```python
from build123d import *

# Parameters (mm, degrees)
BOX268_W                    = 56.5
BOX268_H                    = 56.5
BOX268_DEPTH                = 2
CYLINDER687_R               = 1.5
CYLINDER687_DEPTH           = 20
CYLINDER686_R               = 1.5
CYLINDER686_DEPTH           = 20
COMPOUND411_PLACEMENT_ANGLE = 90
BOX266_W                    = 20
BOX266_H                    = 8
BOX266_DEPTH                = 3
BOX265_W                    = 20
BOX265_H                    = 8
BOX265_DEPTH                = 3
BOX267_W                    = 20
BOX267_H                    = 8
BOX267_DEPTH                = 3
BOX264_W                    = 20
BOX264_H                    = 8
BOX264_DEPTH                = 3
CYLINDER682_R               = 12
CYLINDER682_DEPTH           = 20
CYLINDER672_R               = 5
CYLINDER672_DEPTH           = 4
CYLINDER670_R               = 5
CYLINDER670_DEPTH           = 4
CYLINDER674_R               = 5
CYLINDER674_DEPTH           = 4
CYLINDER675_R               = 5
CYLINDER675_DEPTH           = 4
CYLINDER683_R               = 2.5
CYLINDER683_DEPTH           = 20
CYLINDER673_R               = 2.5
CYLINDER673_DEPTH           = 20
CYLINDER676_R               = 2.5
CYLINDER676_DEPTH           = 20
CYLINDER684_R               = 2.5
CYLINDER684_DEPTH           = 20
CYLINDER681_R               = 3
CYLINDER681_DEPTH           = 5
CYLINDER681_PLACEMENT_ANGLE = 22.5
CYLINDER669_R               = 3
CYLINDER669_DEPTH           = 5
CYLINDER669_PLACEMENT_ANGLE = 67.5
CYLINDER680_R               = 3
CYLINDER680_DEPTH           = 5
CYLINDER680_PLACEMENT_ANGLE = 202.5
CYLINDER677_R               = 3
CYLINDER677_DEPTH           = 5
CYLINDER677_PLACEMENT_ANGLE = 112.5
COMPOUND408_PLACEMENT_ANGLE = 45
CYLINDER679_R               = 1.5
CYLINDER679_DEPTH           = 30
CYLINDER679_PLACEMENT_ANGLE = 22.5
CYLINDER678_R               = 1.5
CYLINDER678_DEPTH           = 30
CYLINDER678_PLACEMENT_ANGLE = 67.5
CYLINDER685_R               = 1.5
CYLINDER685_DEPTH           = 30
CYLINDER685_PLACEMENT_ANGLE = 202.5
CYLINDER671_R               = 1.5
CYLINDER671_DEPTH           = 30
CYLINDER671_PLACEMENT_ANGLE = 112.5
COMPOUND409_PLACEMENT_ANGLE = 45
BOX263_W                    = 68
BOX263_H                    = 64
BOX263_DEPTH                = 8


with BuildPart() as krychle268:
    # Box268 → Box268 (new body)
    with BuildSketch(Plane(origin=(-28.25, -28.25, -68), x_dir=(1, 0, 0), z_dir=(0, 0, 1))):
        with Locations((28.25, 28.25)):
            Rectangle(BOX268_W, BOX268_H)
    extrude(amount=BOX268_DEPTH)


with BuildPart() as obj1:
    # Cylinder687 → Cylinder687 (new body)
    with BuildSketch(Plane(origin=(15.75, 114, 59.48), x_dir=(-1, 0, 0), z_dir=(0, 1, 0))):
        Circle(CYLINDER687_R)
    extrude(amount=CYLINDER687_DEPTH)


with BuildPart() as compound411:
    # Cylinder686 → Cylinder686 (new body)
    with BuildSketch(Plane(origin=(15.75, 114, 38.52), x_dir=(-1, 0, 0), z_dir=(0, 1, 0))):
        Circle(CYLINDER686_R)
    extrude(amount=CYLINDER686_DEPTH)

    # Compound411: union obj1
    add(obj1.part)


with BuildPart() as compound411_1:
    # Compound411 placement: moved
    add(compound411.part.moved(Location((0, 49, -200))).rotate(Axis((0, 49, -200), (1, 0, 0)), COMPOUND411_PLACEMENT_ANGLE))


with BuildPart() as krychle266:
    # Box266 → Box266 (new body)
    with BuildSketch(Plane(origin=(17.55, -27.55, 31), x_dir=(1, 0, 0), z_dir=(0, 0, 1))):
        with Locations((10, 4)):
            Rectangle(BOX266_W, BOX266_H)
    extrude(amount=BOX266_DEPTH)


with BuildPart() as krychle265:
    # Box265 → Box265 (new body)
    with BuildSketch(Plane(origin=(-37.45, 19.55, 31), x_dir=(1, 0, 0), z_dir=(0, 0, 1))):
        with Locations((10, 4)):
            Rectangle(BOX265_W, BOX265_H)
    extrude(amount=BOX265_DEPTH)


with BuildPart() as krychle267:
    # Box267 → Box267 (new body)
    with BuildSketch(Plane(origin=(-37.45, -27.55, 31), x_dir=(1, 0, 0), z_dir=(0, 0, 1))):
        with Locations((10, 4)):
            Rectangle(BOX267_W, BOX267_H)
    extrude(amount=BOX267_DEPTH)


with BuildPart() as compound410:
    # Box264 → Box264 (new body)
    with BuildSketch(Plane(origin=(17.55, 19.55, 31), x_dir=(1, 0, 0), z_dir=(0, 0, 1))):
        with Locations((10, 4)):
            Rectangle(BOX264_W, BOX264_H)
    extrude(amount=BOX264_DEPTH)

    # Compound410: union Krychle266, Krychle265, Krychle267
    add(krychle266.part)
    add(krychle265.part)
    add(krychle267.part)


with BuildPart() as compound410_1:
    # Compound410 placement: moved
    add(compound410.part.moved(Location((0, 0, -4))))


with BuildPart() as obj2:
    # Cylinder682 → Cylinder682 (new body)
    with BuildSketch(Plane.XY.offset(15)):
        Circle(CYLINDER682_R)
    extrude(amount=CYLINDER682_DEPTH)


with BuildPart() as obj3:
    # Cylinder672 → Cylinder672 (new body)
    with BuildSketch(Plane(origin=(23.55, 23.55, 26), x_dir=(1, 0, 0), z_dir=(0, 0, 1))):
        Circle(CYLINDER672_R)
    extrude(amount=CYLINDER672_DEPTH)


with BuildPart() as obj4:
    # Cylinder670 → Cylinder670 (new body)
    with BuildSketch(Plane(origin=(23.55, -23.55, 26), x_dir=(1, 0, 0), z_dir=(0, 0, 1))):
        Circle(CYLINDER670_R)
    extrude(amount=CYLINDER670_DEPTH)


with BuildPart() as obj5:
    # Cylinder674 → Cylinder674 (new body)
    with BuildSketch(Plane(origin=(-23.55, 23.55, 26), x_dir=(1, 0, 0), z_dir=(0, 0, 1))):
        Circle(CYLINDER674_R)
    extrude(amount=CYLINDER674_DEPTH)


with BuildPart() as compound406:
    # Cylinder675 → Cylinder675 (new body)
    with BuildSketch(Plane(origin=(-23.55, -23.55, 26), x_dir=(1, 0, 0), z_dir=(0, 0, 1))):
        Circle(CYLINDER675_R)
    extrude(amount=CYLINDER675_DEPTH)

    # Compound406: union obj3, obj4, obj5
    add(obj3.part)
    add(obj4.part)
    add(obj5.part)


with BuildPart() as compound406_1:
    # Compound406 placement: moved
    add(compound406.part.moved(Location((0, 0, -50))))


with BuildPart() as obj6:
    # Cylinder683 → Cylinder683 (new body)
    with BuildSketch(Plane(origin=(-23.55, 23.55, 20), x_dir=(1, 0, 0), z_dir=(0, 0, 1))):
        Circle(CYLINDER683_R)
    extrude(amount=CYLINDER683_DEPTH)


with BuildPart() as obj7:
    # Cylinder673 → Cylinder673 (new body)
    with BuildSketch(Plane(origin=(-23.55, -23.55, 20), x_dir=(1, 0, 0), z_dir=(0, 0, 1))):
        Circle(CYLINDER673_R)
    extrude(amount=CYLINDER673_DEPTH)


with BuildPart() as obj8:
    # Cylinder676 → Cylinder676 (new body)
    with BuildSketch(Plane(origin=(23.55, -23.55, 20), x_dir=(1, 0, 0), z_dir=(0, 0, 1))):
        Circle(CYLINDER676_R)
    extrude(amount=CYLINDER676_DEPTH)


with BuildPart() as compound407:
    # Cylinder684 → Cylinder684 (new body)
    with BuildSketch(Plane(origin=(23.55, 23.55, 20), x_dir=(1, 0, 0), z_dir=(0, 0, 1))):
        Circle(CYLINDER684_R)
    extrude(amount=CYLINDER684_DEPTH)

    # Compound407: union obj6, obj7, obj8
    add(obj6.part)
    add(obj7.part)
    add(obj8.part)


with BuildPart() as obj9:
    # Cylinder681 → Cylinder681 (new body)
    with BuildSketch(Plane.XY):
        Circle(CYLINDER681_R)
    extrude(amount=CYLINDER681_DEPTH)


with BuildPart() as obj9_1:
    # Cylinder681 placement: moved
    add(obj9.part.moved(Location((-16, 0, 2))).rotate(Axis((-16, 0, 2), (0, 0, 1)), CYLINDER681_PLACEMENT_ANGLE))


with BuildPart() as obj10:
    # Cylinder669 → Cylinder669 (new body)
    with BuildSketch(Plane.XY):
        Circle(CYLINDER669_R)
    extrude(amount=CYLINDER669_DEPTH)


with BuildPart() as obj10_1:
    # Cylinder669 placement: moved
    add(obj10.part.moved(Location((0, 16, 2))).rotate(Axis((0, 16, 2), (0, 0, -1)), CYLINDER669_PLACEMENT_ANGLE))


with BuildPart() as obj11:
    # Cylinder680 → Cylinder680 (new body)
    with BuildSketch(Plane.XY):
        Circle(CYLINDER680_R)
    extrude(amount=CYLINDER680_DEPTH)


with BuildPart() as obj11_1:
    # Cylinder680 placement: moved
    add(obj11.part.moved(Location((16, 0, 2))).rotate(Axis((16, 0, 2), (0, 0, 1)), CYLINDER680_PLACEMENT_ANGLE))


with BuildPart() as compound408:
    # Cylinder677 → Cylinder677 (new body)
    with BuildSketch(Plane.XY):
        Circle(CYLINDER677_R)
    extrude(amount=CYLINDER677_DEPTH)


with BuildPart() as compound408_1:
    # Cylinder677 placement: moved
    add(compound408.part.moved(Location((0, -16, 2))).rotate(Axis((0, -16, 2), (0, 0, 1)), CYLINDER677_PLACEMENT_ANGLE))

    # Compound408: union obj9, obj10, obj11
    add(obj9_1.part)
    add(obj10_1.part)
    add(obj11_1.part)


with BuildPart() as compound408_2:
    # Compound408 placement: moved
    add(compound408_1.part.moved(Location((0, 0, 27))).rotate(Axis((0, 0, 27), (0, 0, 1)), COMPOUND408_PLACEMENT_ANGLE))


with BuildPart() as obj12:
    # Cylinder679 → Cylinder679 (new body)
    with BuildSketch(Plane.XY):
        Circle(CYLINDER679_R)
    extrude(amount=CYLINDER679_DEPTH)


with BuildPart() as obj12_1:
    # Cylinder679 placement: moved
    add(obj12.part.moved(Location((-16, 0, 2))).rotate(Axis((-16, 0, 2), (0, 0, 1)), CYLINDER679_PLACEMENT_ANGLE))


with BuildPart() as obj13:
    # Cylinder678 → Cylinder678 (new body)
    with BuildSketch(Plane.XY):
        Circle(CYLINDER678_R)
    extrude(amount=CYLINDER678_DEPTH)


with BuildPart() as obj13_1:
    # Cylinder678 placement: moved
    add(obj13.part.moved(Location((0, 16, 2))).rotate(Axis((0, 16, 2), (0, 0, -1)), CYLINDER678_PLACEMENT_ANGLE))


with BuildPart() as obj14:
    # Cylinder685 → Cylinder685 (new body)
    with BuildSketch(Plane.XY):
        Circle(CYLINDER685_R)
    extrude(amount=CYLINDER685_DEPTH)


with BuildPart() as obj14_1:
    # Cylinder685 placement: moved
    add(obj14.part.moved(Location((16, 0, 2))).rotate(Axis((16, 0, 2), (0, 0, 1)), CYLINDER685_PLACEMENT_ANGLE))


with BuildPart() as compound409:
    # Cylinder671 → Cylinder671 (new body)
    with BuildSketch(Plane.XY):
        Circle(CYLINDER671_R)
    extrude(amount=CYLINDER671_DEPTH)


with BuildPart() as compound409_1:
    # Cylinder671 placement: moved
    add(compound409.part.moved(Location((0, -16, 2))).rotate(Axis((0, -16, 2), (0, 0, 1)), CYLINDER671_PLACEMENT_ANGLE))

    # Compound409: union obj12, obj13, obj14
    add(obj12_1.part)
    add(obj13_1.part)
    add(obj14_1.part)


with BuildPart() as compound409_2:
    # Compound409 placement: moved
    add(compound409_1.part.moved(Location((0, 0, 14))).rotate(Axis((0, 0, 14), (0, 0, 1)), COMPOUND409_PLACEMENT_ANGLE))


with BuildPart() as common001:
    # Box263 → Box263 (new body)
    with BuildSketch(Plane(origin=(-34, -32, 26), x_dir=(1, 0, 0), z_dir=(0, 0, 1))):
        with Locations((34, 32)):
            Rectangle(BOX263_W, BOX263_H)
    extrude(amount=BOX263_DEPTH)

    # Cut271: cut Compound409
    add(compound409_2.part, mode=Mode.SUBTRACT)

    # Cut270: cut Compound408
    add(compound408_2.part, mode=Mode.SUBTRACT)

    # Cut272: cut Compound407
    add(compound407.part, mode=Mode.SUBTRACT)

    # Cut269: cut Compound406
    add(compound406_1.part, mode=Mode.SUBTRACT)

    # Cut268: cut obj2
    add(obj2.part, mode=Mode.SUBTRACT)

    # Cut267: cut Compound410
    add(compound410_1.part, mode=Mode.SUBTRACT)


with BuildPart() as common001_1:
    # Cut267 placement: moved
    add(common001.part.moved(Location((0, 0, -100))))

    # Cut: cut Compound411
    add(compound411_1.part, mode=Mode.SUBTRACT)

    # Common001: intersect Krychle268
    add(krychle268.part, mode=Mode.INTERSECT)


solid = common001_1.part
```
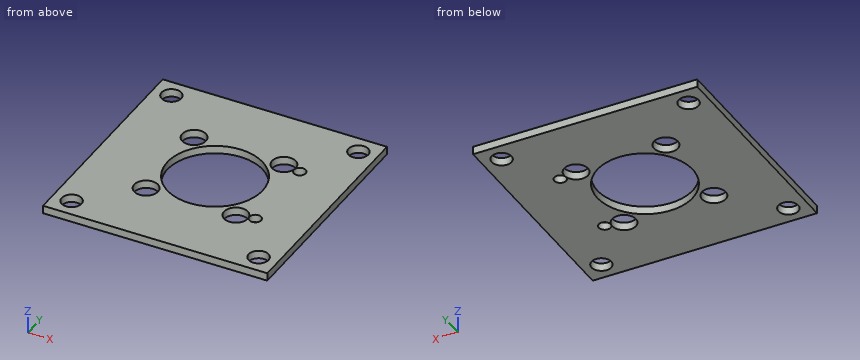
The model under review builds one solid part; all positions refer to its coordinate system, in mm. Give positions to 0.01 mm unless a question says otherwise; leave off trailing zeros. Write each loop counter-clockwise with the first axis right and the second up, starting at its lowest first coordinate (ties: lowest second). Pieces come first, ordered by that corner, then holes. Notation, with made-up numbers: M -29,-18.75 L 27,-18.75 A15 ccw 27,-7.75 Z; hole C -22,-10.75 d8. An arc over 180 degrees is marked long. Answer in a Markdown table with one row per item.
Item 1: Add section C-C on y = -3.5. Give the boundary of the cut face in (x, z).
Check sheet entries:
| item | result |
|---|---|
| outline | M -28.25,-68 L -11.48,-68 L -11.48,-66 L -28.25,-66 Z; M 11.48,-68 L 28.25,-68 L 28.25,-66 L 11.48,-66 Z |
Item 2: Add section D-D on z = -66.95. State how many separate pieces and enclosed holes the cut face has, plus the area to 3 significant figures.
Check sheet entries:
| item | result |
|---|---|
| separate pieces | 1 |
| enclosed holes | 11 |
| area | 2,530 mm2 |
Item 3: Add section A-A on y = -23.55. Give the boundary of the cut face in (x, z).
Check sheet entries:
| item | result |
|---|---|
| outline | M -28.25,-68 L -26.05,-68 L -26.05,-66 L -28.25,-66 Z; M -21.05,-68 L 21.05,-68 L 21.05,-66 L -21.05,-66 Z; M 26.05,-68 L 28.25,-68 L 28.25,-66 L 26.05,-66 Z |
Item 4: For line 1 along Y through (x, z) = (-23.55, -66.85); line 2 along Y through (x, z) = (15.75, -67.5), list the stretches that pass through material, from the lowest coordinate up.
Check sheet entries:
| item | result |
|---|---|
| line 1 | -28.25 to -26.05, -21.05 to 21.05, 26.05 to 28.25 |
| line 2 | -28.25 to -11.98, -8.98 to 8.98, 11.98 to 28.25 |
